```python
from build123d import *

# Parameters (mm, degrees)
SKETCH2_W           = 215
SKETCH2_H           = 30
BOSS_EXTRUDE1_DEPTH = 3.5
SKETCH4_W           = 30
SKETCH4_H           = 8
SKETCH4_W_2         = 40
BOSS_EXTRUDE2_DEPTH = 30
SKETCH5_R           = 8.1
BEARING_HOLES_DEPTH = 6
SKETCH7_R           = 7
CUT_EXTRUDE2_DEPTH  = 116.128189424
FILLET1_R           = 10
HOLES_TBD_R         = 1.65
CUT_EXTRUDE1_DEPTH  = 113.611056296
SKETCH6_W           = 15
SKETCH6_H           = 10
BOSS_EXTRUDE3_DEPTH = 3


with BuildPart() as part:
    # Sketch2 → Boss-Extrude1 (new body)
    with BuildSketch(Plane(origin=(0, 0, 0), x_dir=(1, 0, 0), z_dir=(0, 1, 0))):
        Rectangle(SKETCH2_W, SKETCH2_H)
    extrude(amount=BOSS_EXTRUDE1_DEPTH)

    # Sketch4 → Boss-Extrude2 (add)
    with BuildSketch(Plane(origin=(0, 3.5, 0), x_dir=(1, 0, 0), z_dir=(0, 1, 0))):
        with Locations((92.5, -11)):
            Rectangle(SKETCH4_W, SKETCH4_H)
        with Locations((0, -11)):
            Rectangle(SKETCH4_W_2, SKETCH4_H)
        with Locations((0, 11)):
            Rectangle(SKETCH4_W_2, SKETCH4_H)
        with Locations((92.5, 11)):
            Rectangle(SKETCH4_W, SKETCH4_H)
    extrude(amount=BOSS_EXTRUDE2_DEPTH)

    # Sketch5 → Bearing holes (cut)
    with BuildSketch(Plane.XY.offset(15)):
        with Locations((0, 18.5)):
            Circle(SKETCH5_R)
        with Locations((95, 18.5)):
            Circle(SKETCH5_R)
    bearing_holes = extrude(amount=-BEARING_HOLES_DEPTH, mode=Mode.SUBTRACT)

    # Mirror1: Bearing holes across plane
    add(bearing_holes.mirror(Plane.XY), mode=Mode.SUBTRACT)

    # Sketch7 → Cut-Extrude2 (cut, through all)
    with BuildSketch(Plane.XY.offset(9)):
        with Locations(Location((0, 18.5, 0), (0, 0, 180))):
            Circle(SKETCH7_R)
        with Locations(Location((95, 18.5, 0), (0, 0, 180))):
            Circle(SKETCH7_R)
    extrude(amount=-CUT_EXTRUDE2_DEPTH, mode=Mode.SUBTRACT)

    # Fillet1
    fillet1_edges = [part.edges().sort_by_distance(p)[0] for p in [
        (77.5, 33.5, -11),
        (-20, 33.5, -11),
        (20, 33.5, -11),
        (-20, 33.5, 11),
        (20, 33.5, 11),
        (77.5, 33.5, 11),
    ]]
    fillet(fillet1_edges, radius=FILLET1_R)

    # HOLES TBD → Cut-Extrude1 (cut, through all)
    with BuildSketch(Plane(origin=(0, 3.5, 0), x_dir=(1, 0, 0), z_dir=(0, 1, 0))):
        with Locations(Location((-100, 0, 0), (0, 0, 270))):
            Circle(HOLES_TBD_R)
        with Locations(Location((100, 0, 0), (0, 0, 270))):
            Circle(HOLES_TBD_R)
    extrude(amount=-CUT_EXTRUDE1_DEPTH, mode=Mode.SUBTRACT)

    # Sketch6 → Boss-Extrude3 (add)
    with BuildSketch(Plane(origin=(0, 3.5, 0), x_dir=(1, 0, 0), z_dir=(0, 1, 0))):
        with Locations((-100, 0)):
            Rectangle(SKETCH6_W, SKETCH6_H)
        with Locations((100, 0)):
            Rectangle(SKETCH6_W, SKETCH6_H)
    extrude(amount=BOSS_EXTRUDE3_DEPTH)


solid = part.part
```
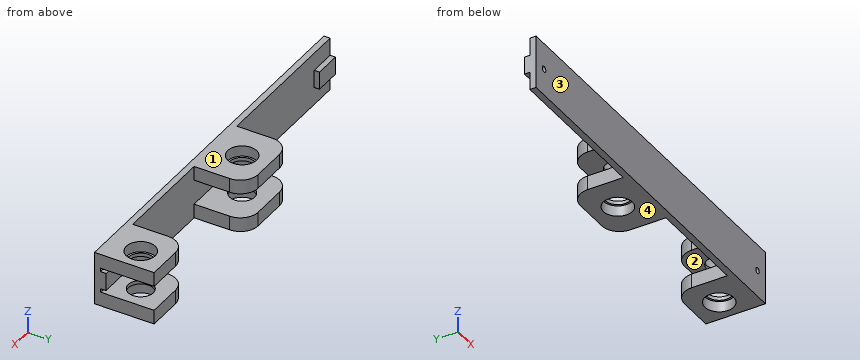
For this review, take the finished solid that the model builds, in its own axes (mm). Face numbers are marked on the shaded views. Coordinates: 2 decimals unless noted, no trailing zeros. Loops run counter-clockwise (first coordinate to the right, second up) from the corner with the lowest first, then second, coordinate; pieces in that order, holes last.
1. Add section D-D, the plane x = 64. Give the boundary of the cut face in (y, z), then the cut area to 3 significant figures.
2. Add section B-B, the plane x = 95. Give the boundary of the cut face in (y, z).
3. Mouldability with a two-part tool opening along Z and no side actions: class the marked faces 1, 2, 3 and 4 as +Z half, -Z half, draft (parallel to the pull), parting line (faces both ways), or undercut.
4. Add section C-C, the plane x = 0. Give the boundary of the cut face in (y, z), then the cut area to 3 significant figures.
5. For line 1 (X direction, y = 18.5, z = 7.85); line 2 (Z direction, x = -14.5, y = 5.5); line 3 (Z direction, x = -5, y = 12.5), list the stretches that pass through material, from the lowest coordinate up.
6. Insertion check: P1, Ø2.5, axis at y = 12.5, z = 10, coming from the -X side; P2, Ø10, axis at x = -69, z = 2.5, coming from the +Y side; P3, Ø5, axis at x = -41, z = 9, coming from the -Y side; P4, Ø5, axis at x = -103.5, z = -1, coming from the +Y side. Each pin has a flat end and moves straight along its axis. Give the tip position at first contact, or say it passes through.
7. Add section A-A, the plane z = 12.5. Give the boundary of the cut face in (x, y).
Result:
1. outline: (0, -15) - (3.5, -15) - (3.5, 15) - (0, 15) - close
1. area: 105 mm2
2. outline: (0, -15) - (10.4, -15) - (10.4, -9) - (11.5, -9) - (11.5, -7) - (3.5, -7) - (3.5, -5) - (6.5, -5) - (6.5, 5) - (3.5, 5) - (3.5, 7) - (11.5, 7) - (11.5, 9) - (10.4, 9) - (10.4, 15) - (0, 15) - close; (25.5, -9) - (26.6, -9) - (26.6, -15) - (33.5, -15) - (33.5, -7) - (25.5, -7) - close; (25.5, 7) - (33.5, 7) - (33.5, 15) - (26.6, 15) - (26.6, 9) - (25.5, 9) - close
3. face 1: +Z half
3. face 2: undercut
3. face 3: draft
3. face 4: -Z half
4. outline: (0, -15) - (10.4, -15) - (10.4, -9) - (11.5, -9) - (11.5, -7) - (3.5, -7) - (3.5, 7) - (11.5, 7) - (11.5, 9) - (10.4, 9) - (10.4, 15) - (0, 15) - close; (25.5, -9) - (26.6, -9) - (26.6, -15) - (33.5, -15) - (33.5, -7) - (25.5, -7) - close; (25.5, 7) - (33.5, 7) - (33.5, 15) - (26.6, 15) - (26.6, 9) - (25.5, 9) - close
4. area: 335 mm2
5. line 1: x = -20 to -7, 7 to 20, 77.5 to 88, 102 to 107.5
5. line 2: z = -15 to -7, 7 to 15
5. line 3: z = -9 to -7, 7 to 9
6. P1: stops at x = -20
6. P2: stops at y = 3.5
6. P3: stops at y = 0
6. P4: stops at y = 6.5
7. outline: (-107.5, 0) - (107.5, 0) - (107.5, 33.5) - (87.5, 33.5) arc R10 ccw to (77.5, 23.5) - (77.5, 3.5) - (20, 3.5) - (20, 23.5) arc R10 ccw to (10, 33.5) - (-10, 33.5) arc R10 ccw to (-20, 23.5) - (-20, 3.5) - (-107.5, 3.5) - close; hole circle Ø16.2 at (0, 18.5); hole circle Ø16.2 at (95, 18.5)
